Here's how the part is built. I have some questions about the finished solid (model axes, mm). Coordinates: 2 decimals unless noted, no trailing zeros. Order: outer loops, then holes, each group sorted by start corner. A loop starts at its lowest first (then second) coordinate and runs counter-clockwise, first axis right, second up. Notation, with made-up numbers: (70, 50.5) - (111, 50.5) arc R12 ccw to (111, 66.5) - close; hole circle Ø4 at (38, 68.5). An arc over 180 degrees is marked (long way). Answer as CSV lines item,"result". Start each with the question number.
Item 1: Imagine slicing it at B-B on y = 12.55. Count the separate pieces of the cut face and the enclosed holes in it, and give its area (3 significant figures).
Item 2: Imagine slicing it at A-A on x = -15.5. List the corners of the cut face in (y, z) for me, and give its area (3 significant figures).
Item 3: I'm going to push flat-ended pins straight in: pin 1 (4 mm diameter, centred on x = 7, y = -10.5, fed in from -Z); pin 2 (4 mm diameter, centred on x = 7, y = -45.55, fed in from +Z). Where does each tip first touch, or does it pass through?
Item 4: I need wall thicknesses on line 1 (Y direction, x = -7, z = 2.6); line 2 (Y direction, x = 7, z = 6.45); line 3 (Y direction, x = 16.5, z = 6). Which ranges of each line are inside material? Lowest first, please.
from build123d import *

# Parameters (mm, degrees)
SKETCH1_W           = 80
SKETCH1_H           = 104
BOSS_EXTRUDE1_DEPTH = 8
SKETCH2_R           = 2.5
CUT_EXTRUDE1_DEPTH  = 8
SKETCH4_R           = 4.25
CUT_EXTRUDE3_DEPTH  = 6
SKETCH5_R           = 1.5
CUT_EXTRUDE4_DEPTH  = 67.090846567
SKETCH6_R           = 2.75
CUT_EXTRUDE5_DEPTH  = 4


with BuildPart() as part:
    # Sketch1 → Boss-Extrude1 (new body)
    with BuildSketch(Plane.XY):
        Rectangle(SKETCH1_W, SKETCH1_H)
    extrude(amount=BOSS_EXTRUDE1_DEPTH)

    # Sketch2 → Cut-Extrude1 (cut)
    with BuildSketch(Plane.XY.offset(8)):
        with Locations((-33, 45.55)):
            Circle(SKETCH2_R)
        with Locations((-7, 45.55)):
            Circle(SKETCH2_R)
        with Locations((-7, 12.55)):
            Circle(SKETCH2_R)
        with Locations((-33, 12.55)):
            Circle(SKETCH2_R)
        with Locations((33, 45.55)):
            Circle(SKETCH2_R)
        with Locations((7, 45.55)):
            Circle(SKETCH2_R)
        with Locations((7, 12.55)):
            Circle(SKETCH2_R)
        with Locations((33, 12.55)):
            Circle(SKETCH2_R)
        with Locations((33, -12.55)):
            Circle(SKETCH2_R)
        with Locations((7, -12.55)):
            Circle(SKETCH2_R)
        with Locations((33, -45.55)):
            Circle(SKETCH2_R)
        with Locations((7, -45.55)):
            Circle(SKETCH2_R)
        with Locations((-7, -45.55)):
            Circle(SKETCH2_R)
        with Locations((-7, -12.55)):
            Circle(SKETCH2_R)
        with Locations((-33, -12.55)):
            Circle(SKETCH2_R)
        with Locations((-33, -45.55)):
            Circle(SKETCH2_R)
    extrude(amount=-CUT_EXTRUDE1_DEPTH, mode=Mode.SUBTRACT)

    # Sketch4 → Cut-Extrude3 (cut)
    with BuildSketch(Plane(origin=(0, 0, 0), x_dir=(-1, 0, 0), z_dir=(0, 0, -1))):
        with Locations((-33, 45.55)):
            Circle(SKETCH4_R)
        with Locations((-7, 45.55)):
            Circle(SKETCH4_R)
        with Locations((-7, 12.55)):
            Circle(SKETCH4_R)
        with Locations((-33, 12.55)):
            Circle(SKETCH4_R)
        with Locations((-33, -12.55)):
            Circle(SKETCH4_R)
        with Locations((-7, -12.55)):
            Circle(SKETCH4_R)
        with Locations((-7, -45.55)):
            Circle(SKETCH4_R)
        with Locations((-33, -45.55)):
            Circle(SKETCH4_R)
        with Locations((7, -45.55)):
            Circle(SKETCH4_R)
        with Locations((33, -45.55)):
            Circle(SKETCH4_R)
        with Locations((7, -12.55)):
            Circle(SKETCH4_R)
        with Locations((33, -12.55)):
            Circle(SKETCH4_R)
        with Locations((7, 12.55)):
            Circle(SKETCH4_R)
        with Locations((33, 12.55)):
            Circle(SKETCH4_R)
        with Locations((7, 45.55)):
            Circle(SKETCH4_R)
        with Locations((33, 45.55)):
            Circle(SKETCH4_R)
    extrude(amount=-CUT_EXTRUDE3_DEPTH, mode=Mode.SUBTRACT)

    # Sketch5 → Cut-Extrude4 (cut, through all)
    with BuildSketch(Plane(origin=(0, 0, 0), x_dir=(-1, 0, 0), z_dir=(0, 0, -1))):
        with Locations((15.5, -15.5)):
            Circle(SKETCH5_R)
        with Locations((-15.5, -15.5)):
            Circle(SKETCH5_R)
        with Locations((-15.5, -46.5)):
            Circle(SKETCH5_R)
        with Locations((15.5, -46.5)):
            Circle(SKETCH5_R)
    extrude(amount=-CUT_EXTRUDE4_DEPTH, mode=Mode.SUBTRACT)

    # Sketch6 → Cut-Extrude5 (cut)
    with BuildSketch(Plane.XY.offset(8)):
        with Locations((15.5, -15.5)):
            Circle(SKETCH6_R)
        with Locations((-15.5, -15.5)):
            Circle(SKETCH6_R)
        with Locations((15.5, -46.5)):
            Circle(SKETCH6_R)
        with Locations((-15.5, -46.5)):
            Circle(SKETCH6_R)
    extrude(amount=-CUT_EXTRUDE5_DEPTH, mode=Mode.SUBTRACT)


solid = part.part
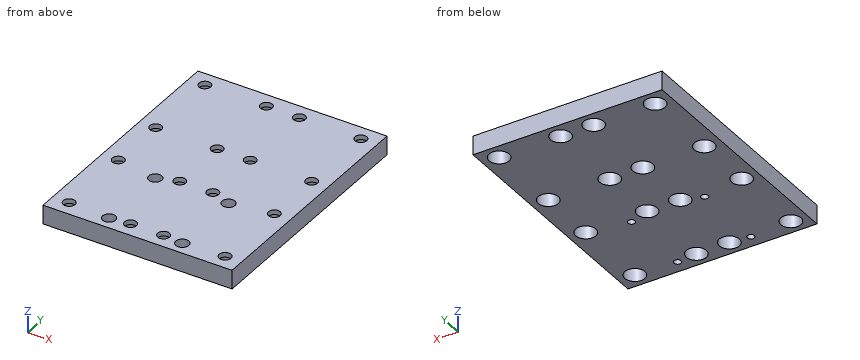
Responses:
1,separate pieces,"5"
1,enclosed holes,"0"
1,area,"396 mm^2"
2,outline,"(-52, 0) - (-48, 0) - (-48, 4) - (-49.25, 4) - (-49.25, 8) - (-52, 8) - close; (-45, 0) - (-17, 0) - (-17, 4) - (-18.25, 4) - (-18.25, 8) - (-43.75, 8) - (-43.75, 4) - (-45, 4) - close; (-14, 0) - (52, 0) - (52, 8) - (-12.75, 8) - (-12.75, 4) - (-14, 4) - close"
2,area,"764 mm^2"
3,pin 1,"stops at z = 6"
3,pin 2,"passes through"
4,line 1,"y = -52 to -49.8, -41.3 to -16.8, -8.3 to 8.3, 16.8 to 41.3, 49.8 to 52"
4,line 2,"y = -52 to -48.05, -43.05 to -15.05, -10.05 to 10.05, 15.05 to 43.05, 48.05 to 52"
4,line 3,"y = -52 to -49.06, -43.94 to -18.06, -12.94 to 52"
